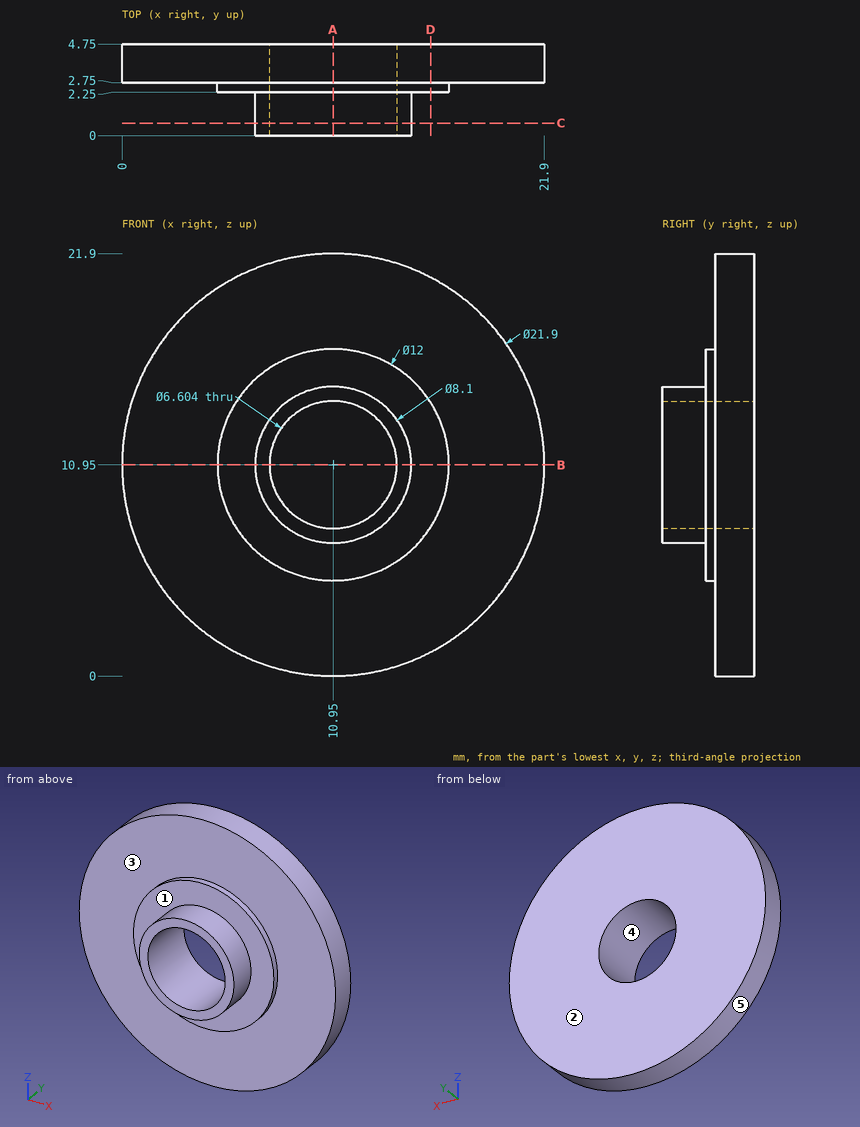
Study the drawing (mm; zero at the part's minimum x, y, z) and answer. A direction names the side the tool comes from. Coordinates: 2 decimals unless noted, no trailing zeros. Loops run counter-clockwise (first coordinate to the right, second up) from the corner with the lowest first, then second, coordinate; pieces in that order, holes last. Notation, with made-up numbers: M 68.5,18.25 L 113.5,18.25 A37 ccw 113.5,54.25 Z; hole C 61,12 d3. An arc over 180 degrees is marked long. Answer in a Markdown table with one row per item.
1) Given pin 1 (1.5 mm diameter, centred on x = 19, y = 3.5, fed in from -Z); pin 2 (6 mm diameter, centred on x = 14, z = 12.5, fed in from -Y); pin 3 (4 mm diameter, centred on x = 6, z = 2.5, fed in from -Y); pin 4 (1.5 mm diameter, centred on x = 16, y = 3.5, fed in from +Z), each flat-ended and moving along its own axis, determine where each tip first touches the part or whether it passes through.
Answers below:
| item | result |
|---|---|
| pin 1 | z = 2.79 |
| pin 2 | y = 0 |
| pin 3 | y = 2.75 |
| pin 4 | z = 21.02 |
2) Find section A-A (x = 10.95). Determine the outline of the cut face in (y, z).
Answers below:
| item | result |
|---|---|
| outline | M 0,6.9 L 2.25,6.9 L 2.25,4.95 L 2.75,4.95 L 2.75,0 L 4.75,0 L 4.75,7.65 L 0,7.65 Z; M 0,14.25 L 4.75,14.25 L 4.75,21.9 L 2.75,21.9 L 2.75,16.95 L 2.25,16.95 L 2.25,15 L 0,15 Z |
3) Find section C-C (y = 0.65). Determine the outline of the cut face in (x, z).
Answers below:
| item | result |
|---|---|
| outline | C 10.95,10.95 d8.1; hole C 10.95,10.95 d6.6 |
4) Find section D-D (x = 16). Determine the outline of the cut face in (y, z), then the cut area to 3 significant figures.
Answers below:
| item | result |
|---|---|
| outline | M 2.25,7.71 L 2.75,7.71 L 2.75,1.23 L 4.75,1.23 L 4.75,20.67 L 2.75,20.67 L 2.75,14.19 L 2.25,14.19 Z |
| area | 42.1 mm^2 |
5) Find the intervals of material crossed by probe 1 along Z at (x, y) = (10.95, 3.1); probe 2 along Z at (x, y) = (10.95, 1.05); probe 3 along X at (y, z) = (0.8, 12.25), in increasing order.
Answers below:
| item | result |
|---|---|
| probe 1 | 0 to 7.65, 14.25 to 21.9 |
| probe 2 | 6.9 to 7.65, 14.25 to 15 |
| probe 3 | 7.11 to 7.91, 13.99 to 14.79 |
6) Determine the mould class of the marked faces 3, 4 and 5 for opening direction Z: released by +Z, released by -Z, zero draft, split by the parting line, or undercut.
Answers below:
| item | result |
|---|---|
| face 3 | zero draft |
| face 4 | undercut |
| face 5 | split by the parting line |
7) Which of the six approach directions +Z, -Z, +X, -X, +Y, -Y give full straight-line access (tool end or side, diameter ignored) to the marked faces 1 and 2?
Answers below:
| item | result |
|---|---|
| face 1 | -Y |
| face 2 | +Z, -Z, +X, -X, +Y |
8) Find section B-B (z = 10.95). Determine the outline of the cut face in (x, y).
Answers below:
| item | result |
|---|---|
| outline | M 0,2.75 L 4.95,2.75 L 4.95,2.25 L 6.9,2.25 L 6.9,0 L 7.65,0 L 7.65,4.75 L 0,4.75 Z; M 14.25,0 L 15,0 L 15,2.25 L 16.95,2.25 L 16.95,2.75 L 21.9,2.75 L 21.9,4.75 L 14.25,4.75 Z |
